Source: CAD feature listing. Evaluate the final solid. Frame: model axes, mm. A direction names the side the tool comes from. Give positions to 0.01 mm unless a question says otherwise; leave off trailing zeros. Write each loop counter-clockwise with the first axis right and the second up, starting at its lowest first coordinate (ties: lowest second). Pieces come first, ordered by that corner, then holes. Notation, with made-up numbers: (24, 40.25) -> (82, 40.25) arc R28 ccw to (82, 76.25) -> close; hole circle Ø6 at (-18.5, -34.75). An arc over 180 degrees is marked (long way). Write item = value, one per line.
from build123d import *

# Parameters (mm, degrees)
SKETCH_3_R          = 9
EXTRUDE_1_DEPTH     = 5
SKETCH_4_R          = 5
CUT_EXTRUDE_1_DEPTH = 8


with BuildPart() as part:
    # 草图2 → 旋转1 (revolve)
    with BuildSketch(Plane.XY):
        Polygon((0, 0), (0, 6.5), (5, 6.5), (5, 3), (10, 3), (10, 0), align=None)
    revolve(axis=Axis((0, 0, 0), (1, 0, 0)))

    # 草图3 → 凸台-拉伸1 (add)
    with BuildSketch(Plane.ZY):
        Circle(SKETCH_3_R)
    extrude(amount=EXTRUDE_1_DEPTH)

    # 草图4 → 切除-拉伸1 (cut)
    with BuildSketch(Plane.ZY.offset(5)):
        Circle(SKETCH_4_R)
    extrude(amount=-CUT_EXTRUDE_1_DEPTH, mode=Mode.SUBTRACT)


solid = part.part
(1) Section query D-D (x = 7). Return loops of the section in (y, z), plus the area to 3 significant figures.
Values follow:
outline = circle Ø6 at (0, 0)
area = 28.3 mm2
(2) Pull-direction query (Z, two-part tool) for faces 4 (the face through (3, 0, 0)), 5 (the face through (5, 3, -1)), 6 (the face through (2.535, -5.158, -3.955)); classes: pulls with the +Z half, pulls with the -Z half, needs draft (parallel to the pull), parting line crosses it, or undercut.
Values follow:
face_4 = undercut
face_5 = needs draft
face_6 = parting line crosses it
(3) Access query for faces 1 (the face through (-2.465, 8.923, -1.172)), 2 (the face through (0, -6, 3)), 3 (the face through (-1.06, -4.88, -1.08)). Directions: +Z, -Z, +X, -X, +Y, -Y. A direction counts if a zero-diameter tool reaches every point of the face in a straight line with its end or side. Return the directions, or none.
Values follow:
face_1 = +X, -X
face_2 = +X
face_3 = -X
(4) First-contact query: pin 1 (10 mm diameter, centred on y = -7, z = -5.5, fed in from +X); pin 2 (1 mm diameter, centred on x = -0.5, y = 3.5, fed in from -Z); pin 3 (3 mm diameter, centred on x = 2, y = -2, fed in from +Z). Flat tips, straight axial feed; report the tip coordinate or a pass-through.
Values follow:
pin_1 = 5
pin_2 = -8.49
pin_3 = 6.48
(5) Material intervals for line 1 (Y direction, x = -3, z = 0); line 2 (Z direction, x = -1.5, y = 0.25); line 3 (X direction, y = -3.75, z = -5), sorted ascending.
Values follow:
line_1 = -9 to -5, 5 to 9
line_2 = -9 to -4.99, 4.99 to 9
line_3 = -5 to 5
(6) Section query B-B (x = 0.75). Return loops of the section in (y, z), plus the area to 3 significant figures.
Values follow:
outline = circle Ø13 at (0, 0); hole circle Ø10 at (0, 0)
area = 54.2 mm2
(7) Section query A-A (y = 0). Return loops of the section in (x, z).
Values follow:
outline = (-5, -9) -> (0, -9) -> (0, -6.5) -> (5, -6.5) -> (5, -3) -> (10, -3) -> (10, 3) -> (5, 3) -> (5, 6.5) -> (0, 6.5) -> (0, 9) -> (-5, 9) -> (-5, 5) -> (3, 5) -> (3, -5) -> (-5, -5) -> close
